Autodesk Inventor part; units mm, degrees
ref_plane "Start plane" through (0, 0, -17.5) normal (0, 0, 1) x (1, 0, 0)
ref_plane "End plane" through (0, 0, 412.5) normal (0, 0, 1) x (1, 0, 0)
ref_plane "Work Plane12" through (0, 180, -17.5) normal (0, 0, -1) x (-1, 0, 0)
ref_plane "Start plane" through (0, 0, -17.5) normal (0, 0, 1) x (1, 0, 0)
ref_plane "End plane" through (0, 0, 412.5) normal (0, 0, 1) x (1, 0, 0)
sketch "Sketch" plane through (0, 0, 0) normal (0, 0, 1) x (1, 0, 0)
  line L0 (-17.5, -13.5) -> (-17.5, 13.5)
  line L1 (-13.5, 17.5) -> (13.5, 17.5)
  line L2 (17.5, 13.5) -> (17.5, -13.5)
  line L3 (13.5, -17.5) -> (-13.5, -17.5)
  arc A0 (-17.5, -13.5) -> (-13.5, -17.5) centre (-13.5, -13.5) ccw
  arc A1 (-13.5, 17.5) -> (-17.5, 13.5) centre (-13.5, 13.5) ccw
  arc A2 (17.5, 13.5) -> (13.5, 17.5) centre (13.5, 13.5) ccw
  arc A3 (13.5, -17.5) -> (17.5, -13.5) centre (13.5, -13.5) ccw
  arc A4 (-13.5, 15.5) -> (-15.5, 13.5) centre (-13.5, 13.5) ccw
  line L4 (-13.5, 15.5) -> (13.5, 15.5)
  arc A5 (15.5, 13.5) -> (13.5, 15.5) centre (13.5, 13.5) ccw
  line L5 (15.5, 13.5) -> (15.5, -13.5)
  arc A6 (13.5, -15.5) -> (15.5, -13.5) centre (13.5, -13.5) ccw
  line L6 (13.5, -15.5) -> (-13.5, -15.5)
  arc A7 (-15.5, -13.5) -> (-13.5, -15.5) centre (-13.5, -13.5) ccw
  line L7 (-15.5, -13.5) -> (-15.5, 13.5)
  line L8 (0, 25.6598) -> (0, -25.6598) construction
  line L9 (-25.6598, 0) -> (25.6598, 0) construction
  dimension "d7" = 4
  dimension "d10" = 35
  dimension "d11" = 35
  dimension "d12" = 2
  dimension "d15" = 17.5
  dimension "d16" = 17.5
extrude "Body" add sketch "Sketch" along normal up to surface (430 mm away) from surface at -17.5
sketch "Sketch3" plane through (0, 0, 0) normal (0, 0, 1) x (1, 0, 0)
  line L0 (0, 0) -> (10, 0)
ref_plane "Work Plane3" through (0, 0, 0) normal (0, -1, 0) x (1, 0, 0)
sketch "Sketch4" plane through (0, 0, 0) normal (0, -1, 0) x (1, 0, 0)
  line L0 (-2, -17.5) -> (12, -17.5)
  line L1 (-2, 412.5) -> (12, 412.5)
  dimension "d18" = 430
ref_plane "Work Plane12" through (0, 180, -17.5) normal (0, 0, -1) x (-1, 0, 0)
split "Split6" plane through (0, 180, -17.5) removes the side toward (0, 0, -1)
ref_plane "Work Plane13" through (17.5, 0, -17.5) normal (-0.7071, 0, -0.7071) x (-0.7071, 0, 0.7071)
split "Split7" plane through (17.5, 0, -17.5) removes the side toward (-0.7071, 0, -0.7071)
ref_plane "Work Plane14" through (17.5, 0, 412.5) normal (-0.7071, 0, 0.7071) x (0.7071, 0, 0.7071)
split "Split8" plane through (17.5, 0, 412.5) removes the side toward (-0.7071, 0, 0.7071)
equation "\"d7\" = G_IR"
equation "\"d10\" = G_H"
equation "\"d11\" = G_W"
equation "\"d12\" = G_T"
equation "\"d15\" = 0.5 * d10"
equation "\"d16\" = 0.5 * d11"
equation "\"d3\" = G_L"
equation "\"G_W\" = 35"
equation "\"G_H\" = 35"
equation "\"G_T\" = 2"
equation "\"G_IR\" = 4"
equation "\"G_L\" = d18"
equation "\"G_OFFSET_START\" = 17.5"
equation "\"G_OFFSET_END\" = 17.5"
equation "\"d13\" = -G_OFFSET_START"
equation "\"d14\" = G_OFFSET_END + B_L"
equation "\"B_L\" = 395"
properties part number "AS 1163 - C350L0 35x35x2.0 SHS - 430" material "Steel, Mild"
Source: CAD feature listing. Evaluate the final solid. Frame: model axes, mm. A direction names the side the tool comes from. Coordinates: 2 decimals unless noted, no trailing zeros. Loops run counter-clockwise (first coordinate to the right, second up) from the corner with the lowest first, then second, coordinate; pieces in that order, holes last. Notation, with made-up numbers: M 22,78 L 33,78 A38 ccw 33,116 Z; hole C 22.25,61 d10. An arc over 180 degrees is marked long. Answer in a Markdown table with one row per item.
Q1. Section C-C on z = 300. Return the cut outline in (x, y), plus the area to 3 significant figures.
Answers below:
| item | result |
|---|---|
| outline | M -17.5,-13.5 A4 ccw -13.5,-17.5 L 13.5,-17.5 A4 ccw 17.5,-13.5 L 17.5,13.5 A4 ccw 13.5,17.5 L -13.5,17.5 A4 ccw -17.5,13.5 Z; hole M -15.5,-13.5 A2 ccw -13.5,-15.5 L 13.5,-15.5 A2 ccw 15.5,-13.5 L 15.5,13.5 A2 ccw 13.5,15.5 L -13.5,15.5 A2 ccw -15.5,13.5 Z |
| area | 254 mm^2 |
Q2. Draft query along Y for faces 3 (the flat face through (-3, 16, 3)), 4 (the flat face through (0, -17.5, 195)), 5 (the flat face through (-15.5, 0, 195)). Return one class per face: pulls with the +Y half, pulls with the -Y half, needs draft (parallel to the pull), parting line crosses it, or undercut.
Answers below:
| item | result |
|---|---|
| face 3 | needs draft |
| face 4 | pulls with the -Y half |
| face 5 | undercut |
Q3. Ray query, probe 1 along Y at (x, z) = (-1, 368.5); probe 2 along Z at (x, y) = (-16, -15). Return the intervals inside material, ascending. Write a range as from..to.
Answers below:
| item | result |
|---|---|
| probe 1 | y = -17.5..-15.5, 15.5..17.5 |
| probe 2 | z = 16..379 |
Q4. Section B-B on y = 7.5. Return the cut outline in (x, z), plus the area to 3 significant figures.
Answers below:
| item | result |
|---|---|
| outline | M -17.5,17.5 L -15.5,15.5 L -15.5,379.5 L -17.5,377.5 Z; M 15.5,-15.5 L 17.5,-17.5 L 17.5,412.5 L 15.5,410.5 Z |
| area | 1,580 mm^2 |
Q5. Set-up query: faces 1 (the flat face through (0, 15.5, 195)), 2 (the flat face through (-3, -16, 392)). Return all of +Z, -Z, +X, -X, +Y, -Y with unobstructed straight access to the full face (end or side cutting, diameter ignored); none if empty.
Answers below:
| item | result |
|---|---|
| face 1 | +Z, -Z |
| face 2 | +Z, -X, +Y, -Y |
Q6. First-contact query: pin 1 (3 mm diameter, centred on x = -13.5, y = -13, fed in from +Z). Flat tip, straight axial feed; report the tip coordinate or a pass-through.
Answers below:
| item | result |
|---|---|
| pin 1 | passes through |
Q7. Section A-A on x = -4. Return the cut outline in (y, z).
Answers below:
| item | result |
|---|---|
| outline | M -17.5,4 L -15.5,4 L -15.5,391 L -17.5,391 Z; M 15.5,4 L 17.5,4 L 17.5,391 L 15.5,391 Z |
